Autodesk Inventor part; units mm, degrees
ref_plane "Slot Start Plane" through (0, 0, -1.7245) normal (0, 0, 1) x (1, 0, 0)
ref_plane "YZ Plane" through (0, 0, 0) normal (1, 0, 0) x (0, 1, 0)
ref_plane "XZ Plane" through (0, 0, 0) normal (0, 1, 0) x (-1, 0, 0)
ref_plane "Slot Start Plane" through (0, 0, -1.7245) normal (0, 0, 1) x (1, 0, 0)
sketch "Key Profile" plane through (0, 0, 0) normal (1, 0, 0) x (0, 1, 0)
  line L0 (-2, 2.8563) -> (0.684, 1.8794)
  arc A0 (1.6188, -1.1745) -> (0.684, 1.8794) centre (0, 0) ccw
  line L1 (-2, 1.3132) -> (0.1881, 0.5168)
  arc A1 (0, -0.55) -> (0.1881, 0.5168) centre (0, 0) ccw
  line L2 (-2, 2.8563) -> (-2, -0.55)
  line L3 (0, 0) -> (-2, 0) construction
  line L4 (0, -0.55) -> (-2, -0.55)
  line L5 (1.6188, -1.1745) -> (-0.097, -0.55)
  line L6 (6, -5.8029) -> (14, 53.1883)
  line L7 (-2, 54.9636) -> (-2, 2.8563)
  arc A2 (14, 53.1883) -> (-2, 54.9636) centre (0, 0) ccw
  line L8 (-2, -0.55) -> (-2, -7.55)
  arc A3 (4, -7.55) -> (6, -5.8029) centre (4, -5.5317) ccw
  line L9 (-2, -7.55) -> (4, -7.55)
  arc A4 (-2, 2.8563) -> (-2, 50.2011) centre (-188.0444, 26.5287) ccw
  point P0 (-0.5, 26.5287)
  dimension "hingeCutRad" = 0.55
  dimension "hingeDepth" = 2
  dimension "d10" = 2
  dimension "keyLength" = 55
  dimension "blackKeyExtraHeight" = 8
  dimension "keyHeight" = 8
  dimension "d107" = 20
  dimension "d122" = 4
  dimension "slotOffset" = 1.1745
  dimension "backWidth" = 7
  dimension "d129" = 4.7625
  dimension "d130" = 1.5
extrude "Key" add sketch "Key Profile" along normal mid plane 9.6 contours A4 L7 A2 L6 A3 L9 L8 L4 L5 A0 L0 | L0 A0 L5 L4 A1 L1 L2
extrude "Protrusion Cutout" cut sketch "Key Profile" along normal mid plane 4.5 contours L0 A0 L5 L4 A1 L1 L2
fillet "Front Fillet" radius 3 1 edges at (0, 14, 53.1883)
sketch "Slot Sketch" plane through (0, 0, -1.7245) normal (0, 0, 1) x (1, 0, 0)
  line L0 (2.15, -2) -> (2.15, 1)
  line L1 (3.1, 4) -> (-3.1, 4)
  line L2 (-2.15, 1) -> (-2.15, -2)
  line L3 (-2.15, -2) -> (2.15, -2)
  line L4 (0, -2) -> (0, 4) construction
  line L5 (-3.1, 4) -> (-3.1, 1)
  line L6 (-3.1, 1) -> (-2.15, 1)
  line L7 (2.15, 1) -> (3.1, 1)
  line L8 (3.1, 1) -> (3.1, 4)
  point P0 (0, 0)
  dimension "d109" = 2
  dimension "slotHeadOffset" = 1
  dimension "slotHeadHeight" = 3
  dimension "slotHeadWidth" = 6.2
  dimension "neckSlotWidth" = 4.3
extrude "Slot" cut sketch "Slot Sketch" against normal through all
fillet "Edge Softening" radius 0.7 10 edges at (4.8, 13.1123, 52.6256) (4.8, 4.6727, 54.8011) (4.8, 5.3278, -7.0517) (4.8, 1, -7.55) (4.8, 9.8172, 22.3446) (-4.8, 5.3278, -7.0517) (-4.8, 1, -7.55) (-4.8, 13.1123, 52.6256) (-4.8, 4.6727, 54.8011) (-4.8, 9.8172, 22.3446)
equation "\"headHeight\" = 3"
equation "\"headOffset\" = 1"
equation "\"keySpacing\" = 0.5"
equation "\"hingeRadTol\" = 0.05"
equation "\"hingeRegRadTol\" = 0.5"
equation "\"hingeRegWidthTol\" = 0.5"
properties part number "BlackKey0" material "PLA Plastic (Black)"
Model file for the job. Use its own axes, mm. A direction names the side the tool comes from. Coordinates: 2 decimals unless noted, no trailing zeros. Order: outer loops, then holes, each group sorted by start corner. A loop starts at its lowest first (then second) coordinate and runs counter-clockwise, first axis right, second up. Notation, with made-up numbers: (-15.75, 45) - (34.25, 45) arc R19 ccw to (34.25, 66) - close; hole circle Ø4 at (-24, 15.25). An arc over 180 degrees is marked (long way). Return JSON: item names as keys, results as strings. Group by question number.
1) Probe line 1 (Z direction, x = -3.5, y = 1.5); line 2 (Y direction, x = -3, z = 4); line 3 (Y direction, x = 2.5, z = 9). List the from-to ranges inside material, lowest first. Write a range as from..to.
2) Saw through at A-A, the plane x = 1. Write the cut outline in (y, z), plus the area to 3 significant figures.
3) Flat gauge pins, fed straight in: P1, Ø1, axis at x = 1.5, y = -1.5, coming from the +Z side; P2, Ø0.8, axis at x = -2.5, z = -5, coming from the +Y side; P3, Ø5, axis at x = -0.5, y = 2, coming from the -Z side; P4, Ø3, axis at x = -0.5, z = 18, coming from the +Y side. Where does each tip first touch, or does it go through?
4) Tool access for faces 1 (the flat face through (-0.031, -0.677, 2.375)), 2 (the flat face through (3.51, -0.92, 0.92)), 3 (the flat face through (3.1, 2, -5)), 4 (the flat face through (-2.15, 0, -5)): list every direction of +Z, -Z, +X, -X, +Y, -Y with a clear straight run to the whole face (end or side of a thin tool).
5) Mould opens along Y. For faces 5 (the flat face through (-0.031, 0.773, -0.867)), 6 (the cylindrical face through (-0.031, 1.905, 0.61)), 7 (the cylindrical face through (-3.543, 0.543, -0.085)), 8 (the cylindrical face through (4.6, 9.66, 22.77)) say: released by +Y, released by -Y, zero draft, split by the parting line, or undercut.
Values found:
{
 "1": {"line 1": "z = -7.55..54.98", "line 2": "y = -1.86..7.33", "line 3": "y = -1.32..8.01"},
 "2": {"outline": "(-2, -1.72) - (4, -1.72) - (4, -7.55) arc R2.02 ccw to (6, -5.8) - (13.63, 50.49) arc R3 ccw to (11.28, 53.83) arc R55 ccw to (-2, 54.96) - (-2, 50.2) arc R187.54 cw to (-2, 2.86) - (0.68, 1.88) arc R2 cw to (1.62, -1.17) - (-0.1, -0.55) - (-2, -0.55) - close", "area": "647 mm²"},
 "3": {"P1": "stops at z = 54.99", "P2": "stops at y = 6.16", "P3": "stops at z = -7.55", "P4": "stops at y = 9.43"},
 "4": {"face 1": "-Y", "face 2": "+X, -X, -Y", "face 3": "-Z", "face 4": "-Z, -Y"},
 "5": {"face 5": "undercut", "face 6": "undercut", "face 7": "released by -Y", "face 8": "released by +Y"}
}
